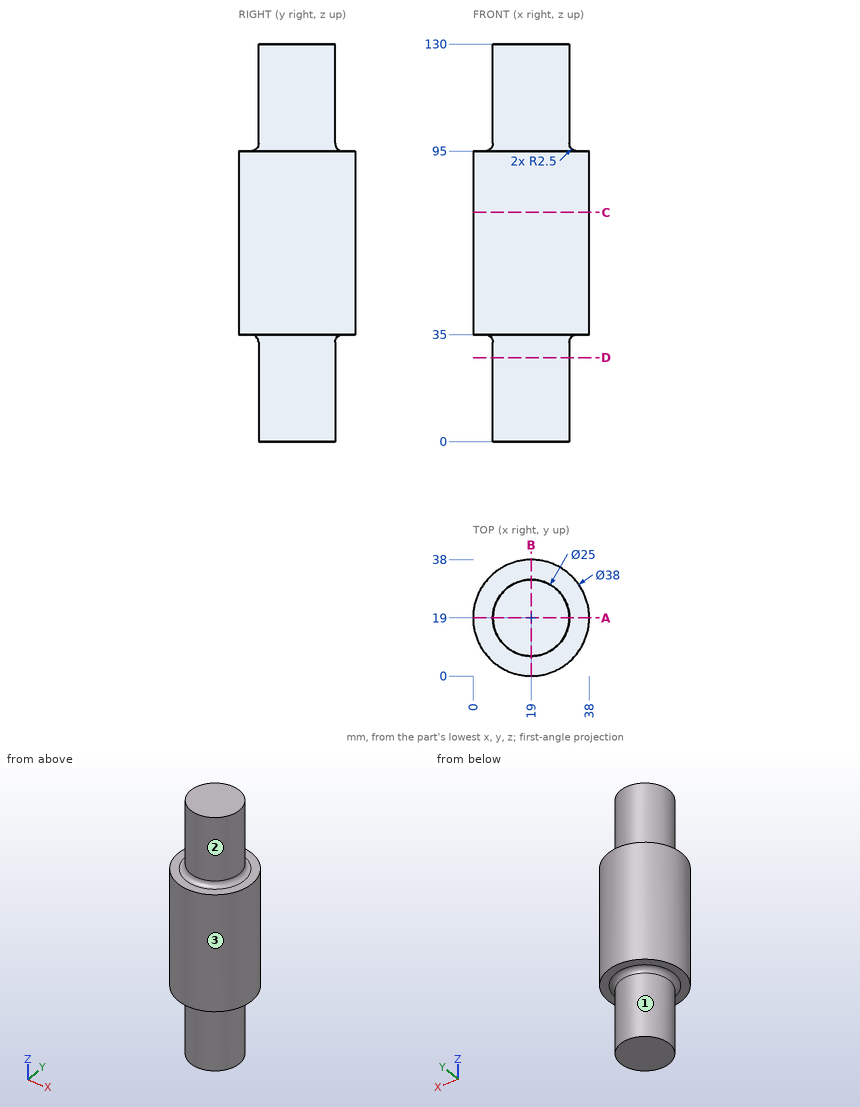
Verification items for this drawing (mm, ordinates from the low corner). A direction names the side the tool comes from. Give positions to 0.01 mm unless a question says otherwise; leave off trailing zeros. Loops run counter-clockwise (first coordinate to the right, second up) from the corner with the lowest first, then second, coordinate; pieces in that order, holes last.
(1) Section check D-D on z = 27.5. Record the cut outline in (x, y), then the cut area to 3 significant figures.
From the geometry:
outline: circle Ø25 at (19, 19)
area: 491 mm2
(2) Set-up check for the marked faces 1, 2 and 3: record each of +Z, -Z, +X, -X, +Y, -Y from which the full face is reachable in a straight line by a thin tool's end or side.
From the geometry:
face 1: -Z
face 2: +Z
face 3: +Z, -Z
(3) Depth check by flat-ended pin: pin 1 Ø2 at (y, z) = (27.5, 65) entering from -X; pin 2 Ø1 at (y, z) = (27, 117) entering from +X; pin 3 Ø4 at (x, z) = (13.5, 13.5) entering from +Y. Enter the tip coordinate at first touch or a pass-through.
From the geometry:
pin 1: stops at x = 1.54
pin 2: stops at x = 29
pin 3: stops at y = 31
(4) Thickness scan on L1, parallel to Z at x = 23.5, y = 33; L2, parallel to X at y = 18, z = 49. Record the ranges inside material, lowest first.
From the geometry:
L1: z = 34.98 to 95.02
L2: x = 0.03 to 37.97
(5) Section check C-C on z = 75. Record the cut outline in (x, y).
From the geometry:
outline: circle Ø38 at (19, 19)
(6) Section check A-A on y = 19. Record the cut outline in (x, z).
From the geometry:
outline: (0, 35) - (4, 35) arc R2.5 cw to (6.5, 32.5) - (6.5, 0) - (31.5, 0) - (31.5, 32.5) arc R2.5 cw to (34, 35) - (38, 35) - (38, 95) - (34, 95) arc R2.5 cw to (31.5, 97.5) - (31.5, 130) - (6.5, 130) - (6.5, 97.5) arc R2.5 cw to (4, 95) - (0, 95) - close
